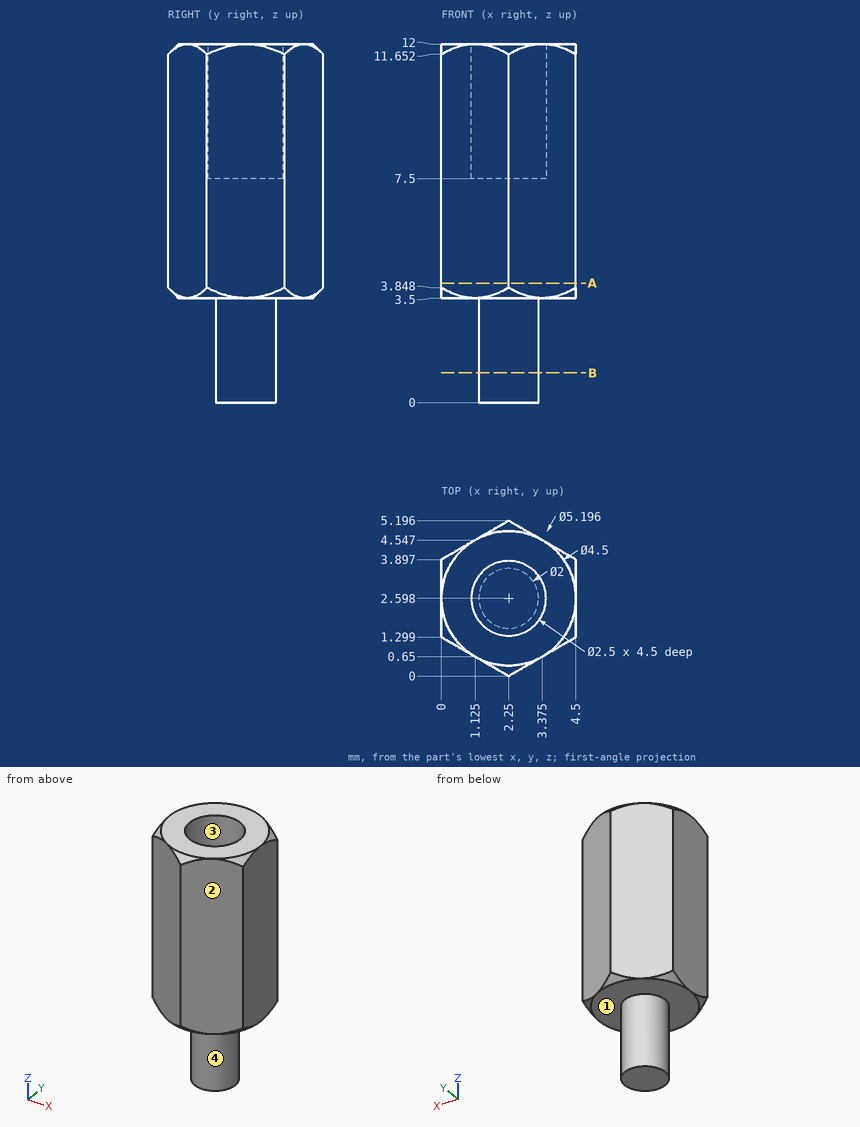
Job drawing, mm, ordinate dimensions from the low corner. One solid piece. Give positions to 0.01 mm unless a question says otherwise; leave off trailing zeros. Write each loop counter-clockwise with the first axis right and the second up, starting at its lowest first coordinate (ties: lowest second). Pieces come first, ordered by that corner, then holes. Notation, with made-up numbers: (78.25, 1.5) -> (133.25, 1.5) arc R35 cw to (133.25, 40.5) -> close; hole circle Ø2 at (41, 25.25). An arc over 180 degrees is marked (long way). Return JSON: item names as keys, results as strings.
Item 1: Drop a flat-ended pin along its axis: pin 1 (1.2 mm diameter, centred on x = 2, y = 3, fed in from +Z). Give the stop position or say it passes through.
Answer below:
{"pin 1": "stops at z = 7.5"}
Item 2: Two-plate mould, pull along Y, no slides. Class the marked faces 1, 2, 3 and 4: +Y half, -Y half, draft (parallel to the pull), parting line (faces both ways), or undercut.
Answer below:
{"face 1": "draft", "face 2": "-Y half", "face 3": "undercut", "face 4": "parting line"}
Item 3: Drill centre lines: probe 1 along Z at (x, y) = (3.2, 1); probe 2 along Z at (x, y) = (1.8, 1.8); probe 3 along X at (y, z) = (3.6, 11.75) (1 decimal). Where is each one in solid material? Low to high.
Answer below:
{"probe 1": "z = 3.5 to 12", "probe 2": "z = 0 to 7.5", "probe 3": "x = 0 to 1.5, 3 to 4.5"}
Item 4: Band-saw the part on B-B (z = 1). List the corners of the cut face in (x, y).
Answer below:
{"outline": "circle Ø2 at (2.25, 2.6)"}
Item 5: Band-saw the part on A-A (z = 4). List the corners of the cut face in (x, y).
Answer below:
{"outline": "(0, 1.3) -> (2.25, 0) -> (4.5, 1.3) -> (4.5, 3.9) -> (2.25, 5.2) -> (0, 3.9) -> close"}
